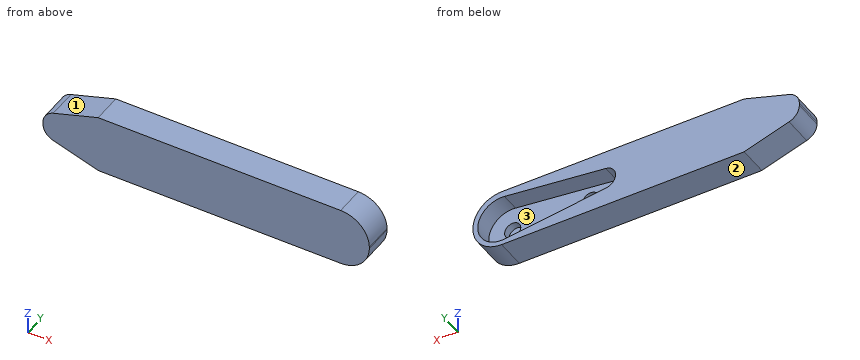
from build123d import *

# Parameters (mm, degrees)
EXTRUDE_1_DEPTH     = 4
CUT_EXTRUDE_1_DEPTH = 2.5
SKETCH_4_R          = 1.1
CUT_EXTRUDE_2_DEPTH = 1


with BuildPart() as part:
    # 草图1 → 凸台-拉伸1 (new body)
    with BuildSketch(Plane(origin=(0, 0, 0), x_dir=(1, 0, 0), z_dir=(0, 1, 0))):
        with BuildLine():
            Line((-22.006488129, 2.068420622), (-15.9, 4))
            Line((-15.9, 4), (17.1, 4))
            ThreePointArc((17.1, 4), (19.857716447, 2.857716447), (21, 0.1))
            Line((21, 0.1), (21, -0.1))
            ThreePointArc((21, -0.1), (19.857716447, -2.857716447), (17.1, -4))
            Line((17.1, -4), (-15.9, -4))
            Line((-15.9, -4), (-22.006488129, -2.068420622))
            ThreePointArc((-22.006488129, -2.068420622), (-23.016748562, -1.343417075), (-23.403312634, -0.161543771))
            Line((-23.403312634, -0.161543771), (-23.403312634, 0.161543771))
            ThreePointArc((-23.403312634, 0.161543771), (-23.016748562, 1.343417075), (-22.006488129, 2.068420622))
        make_face()
    extrude(amount=EXTRUDE_1_DEPTH)

    # 草图2 → 切除-拉伸1 (cut)
    with BuildSketch(Plane(origin=(0, 4, 0), x_dir=(1, 0, 0), z_dir=(0, 1, 0))):
        with BuildLine():
            Line((2.901879582, 1.486858534), (16.670739094, 3.321526824))
            ThreePointArc((16.670739094, 3.321526824), (20.349917095, 0.123213694), (16.716802358, -3.127330099))
            Line((16.716802358, -3.127330099), (2.92313955, -1.489536969))
            ThreePointArc((2.92313955, -1.489536969), (1.600038264, -0.010714012), (2.901879582, 1.486858534))
        make_face()
    extrude(amount=-CUT_EXTRUDE_1_DEPTH, mode=Mode.SUBTRACT)

    # 草图4 → 切除-拉伸2 (cut)
    with BuildSketch(Plane(origin=(0, 1.5, 0), x_dir=(1, 0, 0), z_dir=(0, 1, 0))):
        with Locations((17.1, 0.1)):
            Circle(SKETCH_4_R)
        with Locations((6.5, 0)):
            Circle(SKETCH_4_R)
    extrude(amount=-CUT_EXTRUDE_2_DEPTH, mode=Mode.SUBTRACT)


solid = part.part
Geometry check sheet. Reference: the model listing, model coordinates, mm. Face numbers are marked on the shaded views. Coordinates: 2 decimals unless noted, no trailing zeros. Order: outer loops, then holes, each group sorted by start corner. A loop starts at its lowest first (then second) coordinate and runs counter-clockwise, first axis right, second up. Notation, with made-up numbers: (-24, 44) - (-2, 44) arc R10 ccw to (-2, 52) - close; hole circle Ø11 at (63.5, 7). An arc over 180 degrees is marked (long way). One line per item, written item: value.
(1) Depth check by flat-ended pin: pin 1 Ø3 at (x, z) = (17.1, -0.1) entering from -Y; pin 2 Ø3.5 at (x, z) = (6.5, 0) entering from +Y; pin 3 Ø2 at (y, z) = (2.5, 1.5) entering from +X; pin 4 Ø1.8 at (x, z) = (6.5, 0) entering from +Y. Enter the tip coordinate at first touch or a pass-through.
Data:
pin 1: stops at y = 0
pin 2: stops at y = 1.5
pin 3: stops at x = 20.98
pin 4: stops at y = 0.5
(2) Release check for a two-part mould opening along Z. For the marked faces 1, 2 and 3 record: +Z half, -Z half, draft (parallel to the pull), parting line (faces both ways), or undercut.
Data:
face 1: +Z half
face 2: -Z half
face 3: undercut
(3) Sectioned sample at C-C (x = 5). Enter the section's corners in (y, z), and give its area (3 significant figures).
Data:
outline: (0, -4) - (4, -4) - (4, -1.77) - (1.5, -1.77) - (1.5, 1.74) - (4, 1.74) - (4, 4) - (0, 4) - close
area: 23.2 mm^2
(4) Thickness scan on probe 1 along X at (y, z) = (1, 0); probe 2 along Z at (x, y) = (6.5, 1); probe 3 along Z at (x, y) = (17.1, 0.8). Record the ranges inside material, lowest first. Write a range as from..to.
Data:
probe 1: x = -23.4..5.4, 7.6..16, 18.2..21
probe 2: z = -4..-1.1, 1.1..4
probe 3: z = -4..-1.2, 1..4
(5) Sectioned sample at A-A (y = 3.35). Enter the section's corners in (x, z).
Data:
outline: (-23.4, -0.16) arc R2 ccw to (-22.01, -2.07) - (-15.9, -4) - (17.1, -4) arc R3.9 ccw to (21, -0.1) - (21, 0.1) arc R3.9 ccw to (17.1, 4) - (-15.9, 4) - (-22.01, 2.07) arc R2 ccw to (-23.4, 0.16) - close; hole (2.9, -1.49) - (16.67, -3.32) arc R3.25 ccw (long way) to (16.72, 3.13) - (2.92, 1.49) arc R1.5 ccw to start
(6) Sectioned sample at D-D (z = 2.5). Enter the section's corners in (x, y), and give its area (3 significant figures).
Data:
outline: (-20.64, 0) - (20.17, 0) - (20.17, 4) - (19.05, 4) - (19.05, 1.5) - (11.43, 1.5) - (11.43, 4) - (-20.64, 4) - close
area: 144 mm^2
(7) Sectioned sample at B-B (y = 0.95). Enter the section's corners in (x, z).
Data:
outline: (-23.4, -0.16) arc R2 ccw to (-22.01, -2.07) - (-15.9, -4) - (17.1, -4) arc R3.9 ccw to (21, -0.1) - (21, 0.1) arc R3.9 ccw to (17.1, 4) - (-15.9, 4) - (-22.01, 2.07) arc R2 ccw to (-23.4, 0.16) - close; hole circle Ø2.2 at (6.5, 0); hole circle Ø2.2 at (17.1, -0.1)
